from build123d import *

# Parameters (mm, degrees)
SKETCH_R      = 1.6
PAD_DEPTH     = 1.7
SKETCH001_W   = 10
SKETCH001_H   = 8
SKETCH001_W_2 = 7.5
SKETCH001_H_2 = 6
SKETCH001_W_3 = 13
SKETCH001_H_3 = 13
PAD001_DEPTH  = 12
SKETCH002_R   = 5
PAD002_DEPTH  = 18


with BuildPart() as part:
    # Sketch → Pad (new body)
    with BuildSketch(Plane.XY):
        with BuildLine():
            Line((-21.35, 25.7), (21.35, 25.7))
            ThreePointArc((23.35, 23.7), (22.764214, 25.114214), (21.35, 25.7))
            Line((23.35, 23.7), (23.35, -23.7))
            ThreePointArc((21.35, -25.7), (22.764214, -25.114214), (23.35, -23.7))
            Line((21.35, -25.7), (-21.35, -25.7))
            ThreePointArc((-23.35, -23.7), (-22.764214, -25.114214), (-21.35, -25.7))
            Line((-23.35, -23.7), (-23.35, 23.7))
            ThreePointArc((-21.35, 25.7), (-22.764214, 25.114214), (-23.35, 23.7))
        make_face()
        with Locations((-18.75, -22.2)):
            Circle(SKETCH_R, mode=Mode.SUBTRACT)
        with Locations((18.75, -22.2)):
            Circle(SKETCH_R, mode=Mode.SUBTRACT)
        with Locations((18.75, 22.2)):
            Circle(SKETCH_R, mode=Mode.SUBTRACT)
        with Locations((-18.75, 22.2)):
            Circle(SKETCH_R, mode=Mode.SUBTRACT)
    extrude(amount=PAD_DEPTH)

    # Sketch001 (on Face14 of Pad) → Pad001 (join)
    with BuildSketch(Plane.XY.offset(1.7)):
        with Locations((-6.85, -19.2)):
            Rectangle(SKETCH001_W, SKETCH001_H)
        with Locations((6.15, -19.2)):
            Rectangle(SKETCH001_W, SKETCH001_H)
        with Locations((6.15, 19.2)):
            Rectangle(SKETCH001_W, SKETCH001_H)
        with Locations((-5.6, 19.7)):
            Rectangle(SKETCH001_W_2, SKETCH001_H_2)
        with Locations((-3.85, -5.7)):
            Rectangle(SKETCH001_W_3, SKETCH001_H_3)
    extrude(amount=PAD001_DEPTH)

    # Sketch002 (on Face5 of Pad001) → Pad002 (join)
    with BuildSketch(Plane.XY.offset(1.7)):
        with Locations((-16.85, -9.7)):
            Circle(SKETCH002_R)
        with Locations((-6.35, 9.7)):
            Circle(SKETCH002_R)
    extrude(amount=PAD002_DEPTH)


solid = part.part
Work out the finished part from the listing and answer in its coordinate system (mm). A direction names the side the tool comes from. Give positions to 0.01 mm unless a question says otherwise; leave off trailing zeros. Write each loop counter-clockwise with the first axis right and the second up, starting at its lowest first coordinate (ties: lowest second). Pieces come first, ordered by that corner, then holes. Notation, with made-up numbers: (38, 81) - (67, 81) arc R30 cw to (67, 120) - close; hole circle Ø8 at (-32.75, 31.5). An arc over 180 degrees is marked (long way). One line per item, written item: value. Start each with the question number.
1. Find section A-A (y = -22.2). Write down the section's boundary in (x, z).
2. Find section D-D (y = 20). Write down the section's boundary in (x, z), then the cut area to 3 significant figures.
3. Find section B-B (z = 9.5). Write down the section's boundary in (x, y).
4. For faces 1 (the flat face through (-1.85, 20, 8)), 2 (the flat face through (-7, -19, 13.7)), 3 (the flat face through (-6, 16.7, 8)), 4 (the flat face through (-6, 20, 13.7)), determine the directions among +Z, -Z, +X, -X, +Y, -Y from which every point of the face is accessible in a straight line to the end or side of a thin tool.
5. For a pull along Y with two mould halves and no side action, classify faces 5 (the flat face through (-4, 0.8, 8)), 6 (the flat face through (-10.35, -6, 8)), 7 (the cylindrical face through (22.78, 25.1, 0.84)), 8 (the flat face through (1.15, -19, 8)) as +Y half, -Y half, draft (parallel to the pull), parting line (faces both ways), or undercut.
6. Find section C-C (x = -18.75). Write down the section's boundary in (y, z).
7. Given pin 1 (10 mm diameter, centred on x = 18, y = 8, fed in from -Z); pin 2 (4 mm diameter, centred on x = 8, y = -19, fed in from +Z); pin 3 (1 mm diameter, centred on y = 20, z = 9, fed in from -X); pin 4 (8 mm diameter, centred on x = -17.5, z = 16, fed in from +Y), each flat-ended and moving along its own axis, determine where each tip first touches the part or whether it passes through.
8. Consider probe 1 along Y at (x, z) = (18.75, 0.8); probe 2 along Y at (x, z) = (7, 12.75); probe 3 along Z at (x, y) = (-12, -21.5). Determine where each line is inside the solid, lowest interval first.
Geometry results:
1. outline: (-23.35, 0) - (-20.35, 0) - (-20.35, 1.7) - (-23.35, 1.7) - close; (-17.15, 0) - (17.15, 0) - (17.15, 1.7) - (11.15, 1.7) - (11.15, 13.7) - (1.15, 13.7) - (1.15, 1.7) - (-1.85, 1.7) - (-1.85, 13.7) - (-11.85, 13.7) - (-11.85, 1.7) - (-17.15, 1.7) - close; (20.35, 0) - (23.35, 0) - (23.35, 1.7) - (20.35, 1.7) - close
2. outline: (-23.35, 0) - (23.35, 0) - (23.35, 1.7) - (11.15, 1.7) - (11.15, 13.7) - (1.15, 13.7) - (1.15, 1.7) - (-1.85, 1.7) - (-1.85, 13.7) - (-9.35, 13.7) - (-9.35, 1.7) - (-23.35, 1.7) - close
2. area: 289 mm2
3. outline: circle Ø10 at (-16.85, -9.7); (-11.85, -23.2) - (-1.85, -23.2) - (-1.85, -15.2) - (-11.85, -15.2) - close; circle Ø10 at (-6.35, 9.7); (-10.35, -12.2) - (2.65, -12.2) - (2.65, 0.8) - (-10.35, 0.8) - close; (-9.35, 16.7) - (-1.85, 16.7) - (-1.85, 22.7) - (-9.35, 22.7) - close; (1.15, -23.2) - (11.15, -23.2) - (11.15, -15.2) - (1.15, -15.2) - close; (1.15, 15.2) - (11.15, 15.2) - (11.15, 23.2) - (1.15, 23.2) - close
4. face 1: +Z, +Y
4. face 2: +Z, +X, -X, -Y
4. face 3: +Z, -X
4. face 4: +Z, +X, -X, +Y
5. face 5: undercut
5. face 6: undercut
5. face 7: +Y half
5. face 8: draft
6. outline: (-25.7, 0) - (-23.8, 0) - (-23.8, 1.7) - (-25.7, 1.7) - close; (-20.6, 0) - (20.6, 0) - (20.6, 1.7) - (-5.08, 1.7) - (-5.08, 19.7) - (-14.32, 19.7) - (-14.32, 1.7) - (-20.6, 1.7) - close; (23.8, 0) - (25.7, 0) - (25.7, 1.7) - (23.8, 1.7) - close
7. pin 1: z = 0
7. pin 2: z = 13.7
7. pin 3: x = -9.35
7. pin 4: y = -4.7
8. probe 1: -25.7 to -23.8, -20.6 to 20.6, 23.8 to 25.7
8. probe 2: -23.2 to -15.2, 15.2 to 23.2
8. probe 3: 0 to 1.7
